```python
from build123d import *

# Parameters (mm, degrees)
SKETCH1_W                      = 32
SKETCH1_H                      = 40
BOSS_EXTRUDE1_DEPTH            = 1.6
SKETCH2_R                      = 2.1
CUT_EXTRUDE1_DEPTH             = 52.24997561
LPATTERN1_COUNT                = 3
LPATTERN1_PITCH                = 8
LPATTERN1_COUNT_DIR2           = 5
LPATTERN1_PITCH_DIR2           = 8
EDGE_FLANGE1_STRIP_W           = 8.4
EDGE_FLANGE1_STRIP_H           = 1.6
EDGE_FLANGE1_STRIP_CUT_DEPTH   = 40
EDGE_FLANGE1_STRIP_2_W         = 8.4
EDGE_FLANGE1_STRIP_2_H         = 1.6
EDGE_FLANGE1_STRIP_CUT_2_DEPTH = 40
EDGE_FLANGE1_DEPTH             = 40
EDGE_FLANGE1_BEND_DEPTH        = 40
FILLET1_R                      = 5
SKETCH14_R                     = 2.1
CUT_EXTRUDE2_DEPTH             = 54.23767463
LPATTERN2_COUNT                = 5
LPATTERN2_PITCH                = 8


# Sheet-metal steps are written as plain solids
with BuildPart() as part:
    # Sketch1 → Boss-Extrude1 (new body)
    with BuildSketch(Plane(origin=(0, 0, 0), x_dir=(1, 0, 0), z_dir=(0, 1, 0))):
        with Locations((16, -20)):
            Rectangle(SKETCH1_W, SKETCH1_H)
    extrude(amount=BOSS_EXTRUDE1_DEPTH)

    # Sketch2 → Cut-Extrude1 (cut, through all)
    with BuildSketch(Plane(origin=(0, 1.6, 0), x_dir=(1, 0, 0), z_dir=(0, 1, 0))):
        with Locations(Location((8, -4, 0), (0, 0, 270))):
            Circle(SKETCH2_R)
    cut_extrude1 = extrude(amount=-CUT_EXTRUDE1_DEPTH, mode=Mode.SUBTRACT)

    # LPattern1: Cut-Extrude1 3 × 5
    with Locations(*[(i * LPATTERN1_PITCH, 0, j * LPATTERN1_PITCH_DIR2) for i in range(LPATTERN1_COUNT) for j in range(LPATTERN1_COUNT_DIR2) if (i, j) != (0, 0)]):
        add(cut_extrude1, mode=Mode.SUBTRACT)

    # Edge-Flange1 strip (across the edge) → Edge-Flange1 strip cut (cut)
    with BuildSketch(Plane(origin=(32, 1.6, 40), x_dir=(-1, 0, 0), z_dir=(0, 0, -1))):
        with Locations((-1.6, -0.8)):
            Rectangle(EDGE_FLANGE1_STRIP_W, EDGE_FLANGE1_STRIP_H)
    extrude(amount=EDGE_FLANGE1_STRIP_CUT_DEPTH, mode=Mode.SUBTRACT)

    # Edge-Flange1 strip 2 (across the edge) → Edge-Flange1 strip cut 2 (cut)
    with BuildSketch(Plane(origin=(0, 1.6, 0), x_dir=(1, 0, 0), z_dir=(0, 0, 1))):
        with Locations((-1.6, -0.8)):
            Rectangle(EDGE_FLANGE1_STRIP_2_W, EDGE_FLANGE1_STRIP_2_H)
    extrude(amount=EDGE_FLANGE1_STRIP_CUT_2_DEPTH, mode=Mode.SUBTRACT)

    # Edge-Flange1 section (across the edge) → Edge-Flange1 (add)
    with BuildSketch(Plane(origin=(32, 1.6, 40), x_dir=(-1, 0, 0), z_dir=(0, 0, -1))):
        with BuildLine():
            Line((0, 1), (0, 12.9))
            Line((0, 12.9), (1.6, 12.9))
            Line((1.6, 12.9), (1.6, 1))
            ThreePointArc((1.6, 1), (1.892893219, 0.292893219), (2.6, 0))
            Line((2.6, 0), (2.6, -1.6))
            ThreePointArc((2.6, -1.6), (0.761522369, -0.838477631), (0, 1))
        make_face()
    extrude(amount=EDGE_FLANGE1_DEPTH)

    # Edge-Flange1 section 2 (across the edge) → Edge-Flange1 bend (add)
    with BuildSketch(Plane(origin=(0, 1.6, 0), x_dir=(1, 0, 0), z_dir=(0, 0, 1))):
        with BuildLine():
            Line((0, 1), (0, 12.9))
            Line((0, 12.9), (1.6, 12.9))
            Line((1.6, 12.9), (1.6, 1))
            ThreePointArc((1.6, 1), (1.892893219, 0.292893219), (2.6, 0))
            Line((2.6, 0), (2.6, -1.6))
            ThreePointArc((2.6, -1.6), (0.761522369, -0.838477631), (0, 1))
        make_face()
    extrude(amount=EDGE_FLANGE1_BEND_DEPTH)

    # Fillet1
    fillet1_edges = [part.edges().sort_by_distance(p)[0] for p in [
        (31.2, 14.5, 40),
        (31.2, 14.5, 0),
        (0.8, 14.5, 0),
        (0.8, 14.5, 40),
    ]]
    fillet(fillet1_edges, radius=FILLET1_R)

    # Sketch14 → Cut-Extrude2 (cut, through all)
    with BuildSketch(Plane.ZY):
        with Locations(Location((4, 8.1, 0), (0, 0, 270))):
            Circle(SKETCH14_R)
    cut_extrude2 = extrude(amount=-CUT_EXTRUDE2_DEPTH, mode=Mode.SUBTRACT)

    # LPattern2: Cut-Extrude2 ×5
    with Locations(*[(0, 0, i * LPATTERN2_PITCH) for i in range(1, LPATTERN2_COUNT)]):
        add(cut_extrude2, mode=Mode.SUBTRACT)


solid = part.part
```
Check sheet for the modelled part. Datum: model origin and axes. Units: mm. A direction names the side the tool comes from. Give positions to 0.01 mm unless a question says otherwise; leave off trailing zeros. Loops run counter-clockwise (first coordinate to the right, second up) from the corner with the lowest first, then second, coordinate; pieces in that order, holes last. Notation, with made-up numbers: (-15, 12.25) - (36, 12.25) arc R21 cw to (36, 32.25) - close; hole circle Ø3 at (45, 70). An arc over 180 degrees is marked (long way). One line per question, with ' | ' between items. Start each with the question number.
1. Cross-section at B-B, the plane z = 20. Give the number of separate pieces and of enclosed holes in the cut face, plus the area to 3 significant figures.
2. Material ranges on line 1 along Z through (x, y) = (31.5, 8.1); line 2 along X through (y, z) = (0.6, 28); line 3 along X through (y, z) = (11.5, 7), recorded low to high. Write a range as [from, to].
3. Set-up check for faces 1 (the cylindrical face through (22.722, 0.811, 34.334)), 2 (the cylindrical face through (1.885, 1.901, 19.72)): record each of +Z, -Z, +X, -X, +Y, -Y from which the full face is reachable in a straight line by a thin tool's end or side.
4. Cross-section at C-C, the plane y = 12.75. Enter the section's corners in (x, z), plus the area to 3 significant figures.
5. Gauge pin test, flat ends, axial feed: pin 1 Ø5.5 at (y, z) = (8.1, 20) entering from +X; pin 2 Ø5 at (x, z) = (24, 36) entering from +Y. Record the tip position at first contact, or that the pin passes through.
6. Cross-section at A-A, the plane x = 8. Enter the section's corners in (y, z), plus the area to 3 significant figures.
7. Draft check along X on faces 3 (the cylindrical face through (10.082, 0.811, 11.727)), 4 (the cylindrical face through (31.218, 0.741, 20.28)), 5 (the cylindrical face through (31.19, 10.2, 28.09)). Enter one of: released by +X, released by -X, zero draft, split by the parting line, or undercut.
Check result:
1) separate pieces: 6 | enclosed holes: 0 | area: 56.4 mm2
2) line 1: z = [0, 1.9], [6.1, 9.9], [14.1, 17.9], [22.1, 25.9], [30.1, 33.9], [38.1, 40] | line 2: x = [0.94, 5.9], [10.1, 13.9], [18.1, 21.9], [26.1, 31.06] | line 3: x = [0, 1.6], [30.4, 32]
3) face 1: +Y, -Y | face 2: +Z, -Z, +Y
4) outline: (0, 1.2) - (1.6, 1.2) - (1.6, 38.8) - (0, 38.8) - close; (30.4, 1.2) - (32, 1.2) - (32, 38.8) - (30.4, 38.8) - close | area: 120 mm2
5) pin 1: stops at x = 32 | pin 2: stops at y = 1.6
6) outline: (0, 0) - (1.6, 0) - (1.6, 1.9) - (0, 1.9) - close; (0, 6.1) - (1.6, 6.1) - (1.6, 9.9) - (0, 9.9) - close; (0, 14.1) - (1.6, 14.1) - (1.6, 17.9) - (0, 17.9) - close; (0, 22.1) - (1.6, 22.1) - (1.6, 25.9) - (0, 25.9) - close; (0, 30.1) - (1.6, 30.1) - (1.6, 33.9) - (0, 33.9) - close; (0, 38.1) - (1.6, 38.1) - (1.6, 40) - (0, 40) - close | area: 30.4 mm2
7) face 3: undercut | face 4: released by +X | face 5: zero draft
